```python
from build123d import *

# Parameters (mm, degrees)
F0_W     = 152.5
F0_H     = 92.5
F0_R     = 13.25
F1_DEPTH = 1
F2_DEPTH = 2
F3_R     = 2.55
F4_DEPTH = 2.001


# Not quite as in the source:
# - a feature names something its author has since deleted; it is built from what else it names


with BuildPart() as f1:
    # F0 (on Top) → F1 (new body)
    with BuildSketch(Plane.XY):
        Rectangle(F0_W, F0_H)
        with Locations((-60, -30)):
            Circle(F0_R, mode=Mode.SUBTRACT)
        with Locations((-30, -30)):
            Circle(F0_R, mode=Mode.SUBTRACT)
        with Locations((0, -30)):
            Circle(F0_R, mode=Mode.SUBTRACT)
        with Locations((30, -30)):
            Circle(F0_R, mode=Mode.SUBTRACT)
        with Locations((60, -30)):
            Circle(F0_R, mode=Mode.SUBTRACT)
        with Locations((-60, 0)):
            Circle(F0_R, mode=Mode.SUBTRACT)
        with Locations((-30, 0)):
            Circle(F0_R, mode=Mode.SUBTRACT)
        with Locations((-60, 30)):
            Circle(F0_R, mode=Mode.SUBTRACT)
        with Locations((-30, 30)):
            Circle(F0_R, mode=Mode.SUBTRACT)
        Circle(F0_R, mode=Mode.SUBTRACT)
        with Locations((30, 0)):
            Circle(F0_R, mode=Mode.SUBTRACT)
        with Locations((60, 0)):
            Circle(F0_R, mode=Mode.SUBTRACT)
        with Locations((0, 30)):
            Circle(F0_R, mode=Mode.SUBTRACT)
        with Locations((30, 30)):
            Circle(F0_R, mode=Mode.SUBTRACT)
        with Locations((60, 30)):
            Circle(F0_R, mode=Mode.SUBTRACT)
        with Locations((-60, 30)):
            Circle(F0_R)
        with Locations((-30, 30)):
            Circle(F0_R)
        with Locations((0, 30)):
            Circle(F0_R)
        with Locations((30, 30)):
            Circle(F0_R)
        with Locations((60, 30)):
            Circle(F0_R)
        with Locations((60, 0)):
            Circle(F0_R)
        with Locations((30, 0)):
            Circle(F0_R)
        with Locations((-30, 0)):
            Circle(F0_R)
        with Locations((-60, 0)):
            Circle(F0_R)
        Circle(F0_R)
        with Locations((0, -30)):
            Circle(F0_R)
        with Locations((-30, -30)):
            Circle(F0_R)
        with Locations((-60, -30)):
            Circle(F0_R)
        with Locations((30, -30)):
            Circle(F0_R)
        with Locations((60, -30)):
            Circle(F0_R)
    extrude(amount=F1_DEPTH)

    # F0 (on Top) → F2 (join)
    with BuildSketch(Plane.XY):
        Rectangle(F0_W, F0_H)
        with Locations((-60, -30)):
            Circle(F0_R, mode=Mode.SUBTRACT)
        with Locations((-30, -30)):
            Circle(F0_R, mode=Mode.SUBTRACT)
        with Locations((0, -30)):
            Circle(F0_R, mode=Mode.SUBTRACT)
        with Locations((30, -30)):
            Circle(F0_R, mode=Mode.SUBTRACT)
        with Locations((60, -30)):
            Circle(F0_R, mode=Mode.SUBTRACT)
        with Locations((-60, 0)):
            Circle(F0_R, mode=Mode.SUBTRACT)
        with Locations((-30, 0)):
            Circle(F0_R, mode=Mode.SUBTRACT)
        with Locations((-60, 30)):
            Circle(F0_R, mode=Mode.SUBTRACT)
        with Locations((-30, 30)):
            Circle(F0_R, mode=Mode.SUBTRACT)
        Circle(F0_R, mode=Mode.SUBTRACT)
        with Locations((30, 0)):
            Circle(F0_R, mode=Mode.SUBTRACT)
        with Locations((60, 0)):
            Circle(F0_R, mode=Mode.SUBTRACT)
        with Locations((0, 30)):
            Circle(F0_R, mode=Mode.SUBTRACT)
        with Locations((30, 30)):
            Circle(F0_R, mode=Mode.SUBTRACT)
        with Locations((60, 30)):
            Circle(F0_R, mode=Mode.SUBTRACT)
    extrude(amount=F2_DEPTH)

    # F3 (on face) → F4 (cut, through all)
    with BuildSketch(Plane.XY.offset(2)):
        with Locations((-72.2, 42.2)):
            Circle(F3_R)
        with Locations((72.2, 42.2)):
            Circle(F3_R)
        with Locations((-72.2, -42.2)):
            Circle(F3_R)
        with Locations((72.2, -42.2)):
            Circle(F3_R)
        with Locations((15, -15)):
            Circle(F3_R)
        with Locations((-15, 15)):
            Circle(F3_R)
    extrude(amount=-F4_DEPTH, mode=Mode.SUBTRACT)


solid = f1.part
```
Read the model definition and answer for the solid it produces. Units are mm, in the model's axes. A direction names the side the tool comes from. Round coordinates to 2 decimals unless told otherwise and drop trailing zeros. Loops run counter-clockwise (first coordinate to the right, second up) from the corner with the lowest first, then second, coordinate; pieces in that order, holes last. Notation, with made-up numbers: (44, -14.5) -> (49, -14.5) arc R18 ccw to (49, -1.5) -> close; hole circle Ø4 at (-38, 79). An arc over 180 degrees is marked (long way). One line per item, written item: value.
1) A flat-ended cylindrical pin translates along its axis: P1, Ø21, axis at x = 60, y = 0, coming from the +Z side. Find the tip coordinate at first contact, or state that the pin passes through.
Answer list:
P1: stops at z = 1
2) The mould has two halves that part along X. Classify faces 3 (the face through (-1, 1, 0)), 4 (the face through (-30, 0, 1)): pulls with the +X half, pulls with the -X half, needs draft (parallel to the pull), parting line crosses it, or undercut.
Answer list:
face 3: needs draft
face 4: undercut
3) A cutting plane is placed at D-D (x = 60). Determine the outline of the cut face in (y, z).
Answer list:
outline: (-46.25, 0) -> (46.25, 0) -> (46.25, 2) -> (43.25, 2) -> (43.25, 1) -> (16.75, 1) -> (16.75, 2) -> (13.25, 2) -> (13.25, 1) -> (-13.25, 1) -> (-13.25, 2) -> (-16.75, 2) -> (-16.75, 1) -> (-43.25, 1) -> (-43.25, 2) -> (-46.25, 2) -> close
4) Consider L1, parallel to Y at x = 60.5, z = 1.75; L2, parallel to X at y = -30, z = 1.25; L3, parallel to Y at x = -15, z = 0.95. Determine where each line is inside the solid, lowest interval first. Write a range as [from, to].
Answer list:
L1: y = [-46.25, -43.24], [-16.76, -13.24], [13.24, 16.76], [43.24, 46.25]
L2: x = [-76.25, -73.25], [-46.75, -43.25], [-16.75, -13.25], [13.25, 16.75], [43.25, 46.75], [73.25, 76.25]
L3: y = [-46.25, 12.45], [17.55, 46.25]
5) A cutting plane is placed at A-A (x = 15). Determine the outline of the cut face in (y, z), and give its area (3 significant figures).
Answer list:
outline: (-46.25, 0) -> (-17.55, 0) -> (-17.55, 2) -> (-46.25, 2) -> close; (-12.45, 0) -> (46.25, 0) -> (46.25, 2) -> (-12.45, 2) -> close
area: 175 mm²
6) A cutting plane is placed at C-C (z = 1.5). Give the number of separate pieces and of enclosed holes in the cut face, and give its area (3 significant figures).
Answer list:
separate pieces: 1
enclosed holes: 21
area: 5,710 mm²
7) A cutting plane is placed at B-B (y = -15). Determine the outline of the cut face in (x, z), and give its area (3 significant figures).
Answer list:
outline: (-76.25, 0) -> (12.45, 0) -> (12.45, 2) -> (-76.25, 2) -> close; (17.55, 0) -> (76.25, 0) -> (76.25, 2) -> (17.55, 2) -> close
area: 295 mm²
8) For faces 1 (the face through (-69.844, 41.223, 1.014)), 2 (the face through (46.763, 0.583, 1.493)), determine the directions among +Z, -Z, +X, -X, +Y, -Y from which every point of the face is accessible in a straight line to the end or side of a thin tool.
Answer list:
face 1: +Z, -Z
face 2: +Z
